Autodesk Inventor part; units mm, degrees
ref_plane "YZ Plane" through (0, 0, 0) normal (1, 0, 0) x (0, 1, 0)
ref_plane "XZ Plane" through (0, 0, 0) normal (0, 1, 0) x (-1, 0, 0)
ref_plane "XY Plane" through (0, 0, 0) normal (0, 0, 1) x (1, 0, 0)
sketch "Sketch1" plane through (0, 0, 0) normal (0, 0, 1) x (1, 0, 0)
  line L0 (5, 0) -> (37.3, 0)
  line L1 (42.3, 5) -> (42.3, 37.3)
  line L2 (37.3, 42.3) -> (5, 42.3)
  line L3 (0, 37.3) -> (0, 5)
  line L4 (5, 42.3) -> (0, 37.3)
  line L5 (42.3, 37.3) -> (37.3, 42.3)
  line L6 (37.3, 0) -> (42.3, 5)
  line L7 (0, 5) -> (5, 0)
  point P0 (0, 0)
  point P1 (42.3, 42.3)
  point P2 (42.3, 0)
  point P3 (0, 42.3)
  dimension "d0" = 42.3
  dimension "d1" = 42.3
  dimension "d2" = 5
  dimension "d3" = 5
  dimension "d4" = 5
  dimension "d5" = 5
  dimension "d6" = 5
  dimension "d7" = 5
  dimension "d8" = 5
  dimension "d9" = 5
extrude "Extrusion1" add sketch "Sketch1" along normal blind 38
sketch "Sketch2" plane through (0, 0, 38) normal (0, 0, 1) x (1, 0, 0)
  line L0 (5.65, 36.65) -> (36.65, 36.65) construction
  line L1 (36.65, 36.65) -> (36.65, 5.65) construction
  line L2 (36.65, 5.65) -> (5.65, 5.65) construction
  line L3 (5.65, 5.65) -> (5.65, 36.65) construction
  line L4 (0, 37.3) -> (0, 5)
  line L5 (37.3, 42.3) -> (5, 42.3)
  circle A0 centre (5.65, 36.65) radius 2.25
  circle A1 centre (36.65, 36.65) radius 2.25
  circle A2 centre (36.65, 5.65) radius 2.25
  circle A3 centre (5.65, 5.65) radius 2.25
  point P0 (0, 0)
  point P1 (5.65, 21.15)
  point P2 (0, 21.15)
  point P3 (21.15, 36.65)
  point P4 (21.15, 42.3)
  dimension "d12" = 31
  dimension "d13" = 4.5
extrude "Extrusion2" cut sketch "Sketch2" against normal blind 10
sketch "Sketch3" plane through (0, 0, 38) normal (0, 0, 1) x (1, 0, 0)
  circle A0 centre (21.15, 21.15) radius 11
  line L0 (37.3, 42.3) -> (5, 42.3)
  line L1 (42.3, 5) -> (42.3, 37.3)
  point P0 (0, 0)
  point P1 (21.15, 42.3)
  point P2 (42.3, 21.15)
  dimension "d16" = 22
extrude "Extrusion3" add sketch "Sketch3" along normal blind 2
fillet "Fillet1" radius 1 17 edges at (10.15, 21.15, 40) (21.15, 42.3, 38) (39.8, 39.8, 38) (42.3, 21.15, 38) (39.8, 2.5, 38) (21.15, 0, 38) (2.5, 2.5, 38) (0, 21.15, 38) (2.5, 39.8, 38) (21.15, 42.3, 0) (2.5, 39.8, 0) (39.8, 39.8, 0) (42.3, 21.15, 0) (39.8, 2.5, 0) (21.15, 0, 0) (0, 21.15, 0) (2.5, 2.5, 0)
sketch "Sketch4" plane through (0, 0, 38) normal (0, 0, 1) x (1, 0, 0)
  circle A0 centre (21.15, 21.15) radius 10
  circle A1 centre (21.15, 21.15) radius 2.5
  point P0 (0, 0)
  dimension "d20" = 5
extrude "Extrusion4" add sketch "Sketch4" along normal blind 23.5 contours A1
sketch "Sketch5" plane through (21.15, 21.15, 61.5) normal (0, 0, 1) x (1, 0, 0)
  circle A0 centre (0, 0) radius 2.5
  line L0 (-1.5, 2) -> (1.5, 2)
  circle A1 centre (0, 0) radius 2.5
  point P0 (-21.15, -21.15)
  point P1 (1.5, 2)
  dimension "d23" = 2
extrude "Extrusion5" cut sketch "Sketch5" against normal blind 18 contours L0 A0 picked at (-0.3466, 2.0912)
sketch "Sketch6" plane through (5, 42.3, 1) normal (0, 1, 0) x (1, 0, 0)
  line L0 (32.3, 0) -> (0, 0)
  line L1 (8.05, 0) -> (24.25, 0)
  line L2 (24.25, 0) -> (24.25, -9.4)
  line L3 (24.25, -9.4) -> (8.05, -9.4)
  line L4 (8.05, -9.4) -> (8.05, 0)
  point P0 (-5, 1)
  point P1 (16.15, 0)
  point P2 (24.25, 0)
  dimension "d26" = 16.2
  dimension "d27" = 9.4
extrude "Extrusion6" add sketch "Sketch6" along normal blind 5
properties part number "Motor Model"
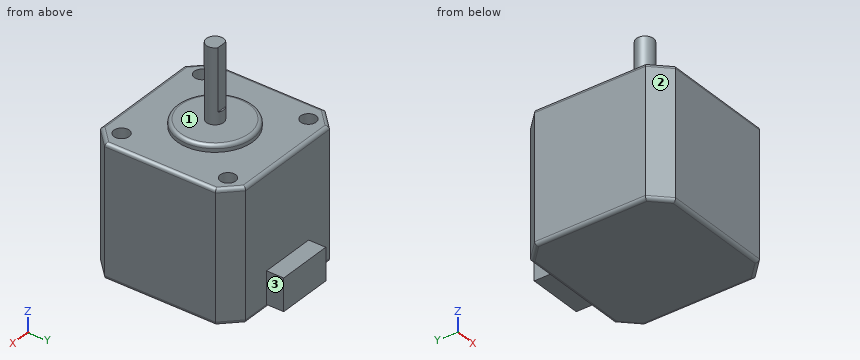
Can you work these out from the model? Positions are in its coordinate system, mm. Face numbers are marked on the shaded views. A direction names the side the tool comes from. Coordinates: 2 decimals unless noted, no trailing zeros. Loops run counter-clockwise (first coordinate to the right, second up) from the corner with the lowest first, then second, coordinate; pieces in that order, holes last.
Item 1: Suppose I cut it at B-B (z = 32). Please give me the cut outline in (x, y).
Answers below:
outline: (0, 5) - (5, 0) - (37.3, 0) - (42.3, 5) - (42.3, 37.3) - (37.3, 42.3) - (5, 42.3) - (0, 37.3) - close; hole circle Ø4.5 at (5.65, 5.65); hole circle Ø4.5 at (5.65, 36.65); hole circle Ø4.5 at (36.65, 5.65); hole circle Ø4.5 at (36.65, 36.65)
Item 2: Suppose I cut it at C-C (y = 21.15). Please give me the cut outline in (x, z).
Answers below:
outline: (0, 1) arc R1 ccw to (1, 0) - (41.3, 0) arc R1 ccw to (42.3, 1) - (42.3, 37) arc R1 ccw to (41.3, 38) - (32.15, 38) - (32.15, 39) arc R1 ccw to (31.15, 40) - (23.65, 40) - (23.65, 61.5) - (18.65, 61.5) - (18.65, 40) - (11.15, 40) arc R1 ccw to (10.15, 39) - (10.15, 38) - (1, 38) arc R1 ccw to (0, 37) - close
Item 3: Suppose I cut it at D-D (z = 20). Please give me the cut outline in (x, y).
Answers below:
outline: (0, 5) - (5, 0) - (37.3, 0) - (42.3, 5) - (42.3, 37.3) - (37.3, 42.3) - (5, 42.3) - (0, 37.3) - close
Item 4: Please list where these lines run through material, in increasing order: L1, parallel to Y at x = 5.65, z = 30.75; L2, parallel to Y at x = 36, z = 32; L3, parallel to Z at x = 16.5, y = 17.
Answers below:
L1: y = 0 to 3.4, 7.9 to 34.4, 38.9 to 42.3
L2: y = 0 to 3.5, 7.8 to 34.5, 38.8 to 42.3
L3: z = 0 to 40
Item 5: Suppose I cut it at A-A (x = 21.15). Please give me the cut outline in (y, z), then the cut area to 3 significant figures.
Answers below:
outline: (0, 1) arc R1 ccw to (1, 0) - (41.3, 0) arc R1 ccw to (42.3, 1) - (47.3, 1) - (47.3, 10.4) - (42.3, 10.4) - (42.3, 37) arc R1 ccw to (41.3, 38) - (32.15, 38) - (32.15, 39) arc R1 ccw to (31.15, 40) - (23.65, 40) - (23.65, 43.5) - (23.15, 43.5) - (23.15, 61.5) - (18.65, 61.5) - (18.65, 40) - (11.15, 40) arc R1 ccw to (10.15, 39) - (10.15, 38) - (1, 38) arc R1 ccw to (0, 37) - close
area: 1,800 mm2
Item 6: Which directions (+Z, -Z, +X, -X, +Y, -Y) give clear straight access to the entire face, cutting with the end or side of a thin tool? Please do the marked faces 1, 2 and 3.
Answers below:
face 1: +Z
face 2: +Z, -Z, -X, -Y
face 3: +Z, -Z, +X, +Y
Item 7: I'm going to push flat-ended pins straight in: pin 1 (6 mm diameter, centred on y = 29.5, z = 40.5, fed in from +X); pin 2 (10 mm diameter, centred on y = 27.5, z = 47, fed in from -X); pin 3 (3.5 mm diameter, centred on x = 36.5, y = 36.5, fed in from +Z). Where does each tip first touch, or does it pass through?
Answers below:
pin 1: stops at x = 42.17
pin 2: stops at x = 19.05
pin 3: stops at z = 28
